Build history of the part. All positions in model axes, mm. Round coordinates to 2 decimals unless told otherwise and drop trailing zeros. Loops run counter-clockwise (first coordinate to the right, second up) from the corner with the lowest first, then second, coordinate; pieces in that order, holes last. Notation, with made-up numbers: M 72,70 L 110,70 A26 ccw 110,92 Z; hole C 3,-19 d10. An arc over 180 degrees is marked long. One line per item, written item: value.
```python
from build123d import *

# Parameters (mm, degrees)
F0_W     = 269.875
F0_H     = 273.05
F1_DEPTH = 19.05
F3_DEPTH = 19.05
F5_DEPTH = 19.05
F7_DEPTH = 19.05
F8_W     = 269.875
F8_H     = 3.175
F9_DEPTH = 19.05


with BuildPart() as f1:
    # F0 (on Top) → F1 (new body)
    with BuildSketch(Plane.XY):
        Rectangle(F0_W, F0_H)
    extrude(amount=F1_DEPTH)

    # F2 (on face) → F3 (cut, through all)
    with BuildSketch(Plane.XY.offset(19.05)):
        with BuildLine():
            ThreePointArc((-106.255823, 57.15), (-84.675295, 85.944848), (-55.5625, 107.094496))
            Line((-55.5625, 107.094496), (-55.5625, 127))
            Line((-55.5625, 127), (-125.4125, 127))
            Line((-125.4125, 127), (-125.4125, 57.15))
            Line((-125.4125, 57.15), (-106.255823, 57.15))
        make_face()
        with BuildLine():
            Line((125.4125, 57.15), (125.4125, 127))
            Line((125.4125, 127), (55.5625, 127))
            Line((55.5625, 127), (55.5625, 107.0864))
            ThreePointArc((55.5625, 107.0864), (84.67437, 85.94048), (106.255823, 57.15))
            Line((106.255823, 57.15), (125.4125, 57.15))
        make_face()
    extrude(amount=-F3_DEPTH, mode=Mode.SUBTRACT)

    # F4 (on face) → F5 (cut, through all)
    with BuildSketch(Plane.XY.offset(19.05)):
        with BuildLine():
            ThreePointArc((-125.4125, -107.445267), (-125.4252, -107.9373), (-125.4125, -108.429333))
            Line((-125.4125, -108.429333), (-125.4125, -107.445267))
        make_face()
        with BuildLine():
            Line((-125.4125, -107.445267), (-125.4125, -108.429333))
            ThreePointArc((-125.4125, -108.429333), (-115.8875, -117.475), (-106.3625, -108.429333))
            Line((-106.3625, -108.429333), (-106.3625, -107.445267))
            Line((-106.3625, -107.445267), (-106.3625, -71.514178))
            ThreePointArc((-106.3625, -71.514178), (-115.8875, -61.453752), (-125.4125, -71.514178))
            Line((-125.4125, -71.514178), (-125.4125, -107.445267))
        make_face()
        with BuildLine():
            Line((-106.3625, -107.445267), (-106.3625, -108.429333))
            ThreePointArc((-106.3625, -108.429333), (-106.3498, -107.9373), (-106.3625, -107.445267))
        make_face()
        with BuildLine():
            Line((106.3625, -71.485033), (106.3625, -70.993))
            Line((106.3625, -70.993), (125.4125, -70.993))
            Line((125.4125, -70.993), (125.4125, -71.485033))
            ThreePointArc((125.4125, -71.485033), (115.8875, -61.4553), (106.3625, -71.485033))
        make_face()
        with BuildLine():
            Line((125.4125, -70.993), (106.3625, -70.993))
            Line((106.3625, -70.993), (106.3625, -71.485033))
            Line((106.3625, -71.485033), (106.3625, -107.445267))
            Line((106.3625, -107.445267), (106.3625, -108.429333))
            ThreePointArc((106.3625, -108.429333), (115.8875, -117.475), (125.4125, -108.429333))
            Line((125.4125, -108.429333), (125.4125, -107.445267))
            Line((125.4125, -107.445267), (125.4125, -71.485033))
            Line((125.4125, -71.485033), (125.4125, -70.993))
        make_face()
        with BuildLine():
            Line((106.3625, -108.429333), (106.3625, -107.445267))
            ThreePointArc((106.3625, -107.445267), (106.3498, -107.9373), (106.3625, -108.429333))
        make_face()
        with BuildLine():
            ThreePointArc((125.4125, -108.429333), (125.4252, -107.9373), (125.4125, -107.445267))
            Line((125.4125, -107.445267), (125.4125, -108.429333))
        make_face()
    extrude(amount=-F5_DEPTH, mode=Mode.SUBTRACT)

    # F6 (on face) → F7 (cut, through all)
    with BuildSketch(Plane.XY.offset(19.05)):
        with BuildLine():
            Line((24.13, -77.47), (24.13, 0))
            ThreePointArc((24.13, 0), (0, 24.13), (-24.13, 0))
            Line((-24.13, 0), (-24.13, -77.47))
            Line((-24.13, -77.47), (24.13, -77.47))
        make_face()
    extrude(amount=-F7_DEPTH, mode=Mode.SUBTRACT)

    # F8 (on face) → F9 (cut, through all)
    with BuildSketch(Plane.XY.offset(19.05)):
        with Locations((0, -134.9375)):
            Rectangle(F8_W, F8_H)
    extrude(amount=-F9_DEPTH, mode=Mode.SUBTRACT)


solid = f1.part
```
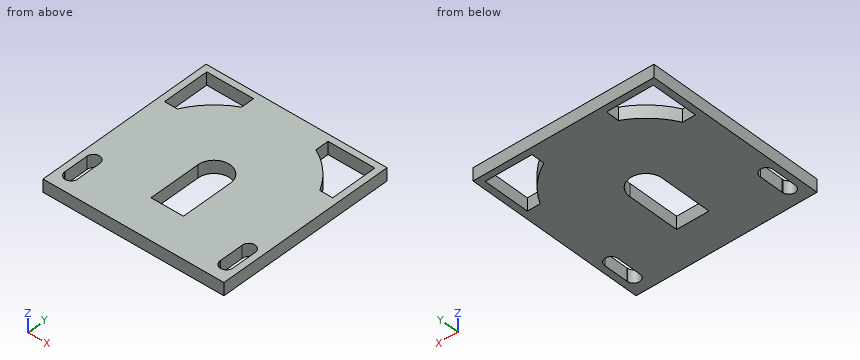
Item 1: Slice it at B-B, the plane x = 0. Give the cut face in (y, z) (3 decimals), and give its area (3 significant figures).
Check values:
outline: M -133.35,0 L -77.47,0 L -77.47,19.05 L -133.35,19.05 Z; M 24.13,0 L 136.525,0 L 136.525,19.05 L 24.13,19.05 Z
area: 3,210 mm2
Item 2: Slice it at A-A, the plane y = 119. Give the cut face in (x, z).
Check values:
outline: M -134.94,0 L -125.41,0 L -125.41,19.05 L -134.94,19.05 Z; M -55.56,0 L 55.56,0 L 55.56,19.05 L -55.56,19.05 Z; M 125.41,0 L 134.94,0 L 134.94,19.05 L 125.41,19.05 Z
Item 3: Slice it at C-C, the plane z = 15.5. Give the number of separate pieces and of enclosed holes in the cut face, and give its area (3 significant figures).
Check values:
separate pieces: 1
enclosed holes: 5
area: 59,500 mm2
Item 4: Slice it at D-D, the plane y = 80. Give the cut face in (x, z).
Check values:
outline: M -134.94,0 L -125.41,0 L -125.41,19.05 L -134.94,19.05 Z; M -90.31,0 L 90.31,0 L 90.31,19.05 L -90.31,19.05 Z; M 125.41,0 L 134.94,0 L 134.94,19.05 L 125.41,19.05 Z
Item 5: Wall check: line 1 along X through (y, z) = (-107, 3); line 2 along X through (y, z) = (115.5, 16.25); line 3 along X through (y, z) = (-51, 2). Give the ranges that are in metal, low to high.
Check values:
line 1: x = -134.94 to -125.41, -106.36 to 106.36, 125.41 to 134.94
line 2: x = -134.94 to -125.41, -55.56 to 55.56, 125.41 to 134.94
line 3: x = -134.94 to -24.13, 24.13 to 134.94
